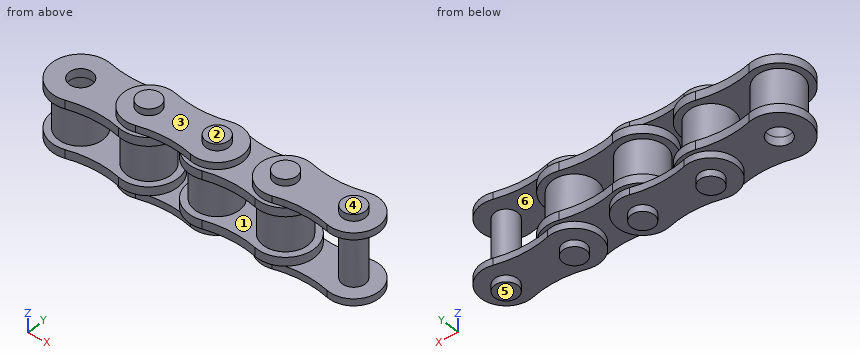
```python
from build123d import *

# Parameters (mm, degrees)
SKETCH4_R                  = 3.175
SKETCH4_R_2                = 1.6637
BOSS_EXTRUDE1_DEPTH        = 2.86
BOSS_EXTRUDE1_2_DEPTH      = 2.86
SKETCH5_R                  = 1.6383
BOSS_EXTRUDE2_DEPTH        = 1.2446
LPATTERN1_COUNT            = 2
LPATTERN1_PITCH            = 9.525
SKETCH7_R                  = 1.6383
BOSS_EXTRUDE3_DEPTH        = 0.9906
BOSS_EXTRUDE4_DEPTH        = 6.096
BOSS_EXTRUDE4_DEPTH_BACK   = 6.096
SKETCH8_R                  = 1.6383
BOSS_EXTRUDE4_2_DEPTH      = 6.096
BOSS_EXTRUDE4_2_DEPTH_BACK = 6.096
LPATTERN2_COUNT            = 2
LPATTERN2_PITCH            = 19.05


with BuildPart() as part:
    # Sketch4 → Boss-Extrude1 (new, symmetric)
    with BuildSketch(Plane.XY):
        with Locations((-4.7625, 0)):
            Circle(SKETCH4_R)
        with Locations((-4.7625, 0)):
            Circle(SKETCH4_R_2, mode=Mode.SUBTRACT)
    extrude(amount=BOSS_EXTRUDE1_DEPTH, both=True)


with BuildPart() as body_2:
    # Sketch4 → Boss-Extrude1 2 (new, symmetric)
    with BuildSketch(Plane.XY):
        with Locations((4.7625, 0)):
            Circle(SKETCH4_R)
        with Locations((4.7625, 0)):
            Circle(SKETCH4_R_2, mode=Mode.SUBTRACT)
    extrude(amount=BOSS_EXTRUDE1_2_DEPTH, both=True)


with BuildPart() as body_3:
    # Sketch5 → Boss-Extrude2 (new body)
    with BuildSketch(Plane.XY.offset(2.86)):
        with BuildLine():
            ThreePointArc((-3.71992076, 3.967398762), (-8.8646, 0), (-3.71992076, -3.967398762))
            ThreePointArc((-3.71992076, -3.967398762), (0, -3.486785), (3.71992076, -3.967398762))
            ThreePointArc((3.71992076, -3.967398762), (8.8646, 0), (3.71992076, 3.967398762))
            ThreePointArc((3.71992076, 3.967398762), (0, 3.486785), (-3.71992076, 3.967398762))
        make_face()
        with Locations((-4.7625, 0)):
            Circle(SKETCH5_R, mode=Mode.SUBTRACT)
        with Locations((4.7625, 0)):
            Circle(SKETCH5_R, mode=Mode.SUBTRACT)
    extrude(amount=BOSS_EXTRUDE2_DEPTH)


with BuildPart() as lpattern1_1:
    # LPattern1: pattern copy
    add(body_2.part.moved(Location(Vector(1, 0, 0) * (1 * LPATTERN1_PITCH))))


with BuildPart() as body_5:
    # Sketch7 → Boss-Extrude3 (new body)
    with BuildSketch(Plane.XY.offset(-4.1554)):
        with BuildLine():
            ThreePointArc((5.704721623, 3.48471247), (1.152652, 0), (5.704721623, -3.48471247))
            ThreePointArc((5.704721623, -3.48471247), (9.525, -2.977345042), (13.345278377, -3.48471247))
            ThreePointArc((13.345278377, -3.48471247), (17.897348, 0), (13.345278377, 3.48471247))
            ThreePointArc((13.345278377, 3.48471247), (9.525, 2.977345042), (5.704721623, 3.48471247))
        make_face()
        with Locations((4.7625, 0)):
            Circle(SKETCH7_R, mode=Mode.SUBTRACT)
        with Locations((14.2875, 0)):
            Circle(SKETCH7_R, mode=Mode.SUBTRACT)
    extrude(amount=-BOSS_EXTRUDE3_DEPTH)


with BuildPart() as body_6:
    # Mirror1: mirrored copy
    add(body_3.part.mirror(Plane.XY))


with BuildPart() as body_7:
    # Mirror1 2: mirrored copy
    add(body_5.part.mirror(Plane.XY))


with BuildPart() as body_8:
    # Sketch8 → Boss-Extrude4 (new, two sides: drawn at the far end of the back side and taken through both)
    with BuildSketch(Plane.XY.offset(-BOSS_EXTRUDE4_DEPTH_BACK)):
        with Locations(Location((4.7625, 0, 0), (0, 0, 180))):
            Circle(SKETCH8_R)
    extrude(amount=BOSS_EXTRUDE4_DEPTH + BOSS_EXTRUDE4_DEPTH_BACK)


with BuildPart() as body_9:
    # Sketch8 → Boss-Extrude4 2 (new, two sides: drawn at the far end of the back side and taken through both)
    with BuildSketch(Plane.XY.offset(-BOSS_EXTRUDE4_2_DEPTH_BACK)):
        with Locations(Location((14.2875, 0, 0), (0, 0, 180))):
            Circle(SKETCH8_R)
    extrude(amount=BOSS_EXTRUDE4_2_DEPTH + BOSS_EXTRUDE4_2_DEPTH_BACK)


with BuildPart() as lpattern2_1:
    # LPattern2: pattern copy
    add(body_9.part.moved(Location(Vector(1, 0, 0) * (1 * LPATTERN2_PITCH))))


with BuildPart() as lpattern2_2:
    # LPattern2: pattern copy
    add(body_8.part.moved(Location(Vector(1, 0, 0) * (1 * LPATTERN2_PITCH))))


with BuildPart() as lpattern2_3:
    # LPattern2: pattern copy
    add(body_7.part.moved(Location(Vector(1, 0, 0) * (1 * LPATTERN2_PITCH))))


with BuildPart() as lpattern2_4:
    # LPattern2: pattern copy
    add(body_6.part.moved(Location(Vector(1, 0, 0) * (1 * LPATTERN2_PITCH))))


with BuildPart() as lpattern2_5:
    # LPattern2: pattern copy
    add(body_5.part.moved(Location(Vector(1, 0, 0) * (1 * LPATTERN2_PITCH))))


with BuildPart() as lpattern2_6:
    # LPattern2: pattern copy
    add(lpattern1_1.part.moved(Location(Vector(1, 0, 0) * (1 * LPATTERN2_PITCH))))


with BuildPart() as lpattern2_7:
    # LPattern2: pattern copy
    add(body_3.part.moved(Location(Vector(1, 0, 0) * (1 * LPATTERN2_PITCH))))


with BuildPart() as lpattern2_8:
    # LPattern2: pattern copy
    add(body_2.part.moved(Location(Vector(1, 0, 0) * (1 * LPATTERN2_PITCH))))


with BuildPart() as lpattern2_9:
    # LPattern2: pattern copy
    add(part.part.moved(Location(Vector(1, 0, 0) * (1 * LPATTERN2_PITCH))))


with BuildPart() as body_2_1:
    add(body_2.part)

    # Combine1: union body 3, LPattern1_1, body 5, body 6, body 7, body 8, body 9, LPattern2_1, LPattern2_2, LPattern2_3, LPattern2_4, LPattern2_5, LPattern2_7, LPattern2_8, LPattern2_9, part
    add(body_3.part)
    add(lpattern1_1.part)
    add(body_5.part)
    add(body_6.part)
    add(body_7.part)
    add(body_8.part)
    add(body_9.part)
    add(lpattern2_1.part)
    add(lpattern2_2.part)
    add(lpattern2_3.part)
    add(lpattern2_4.part)
    add(lpattern2_5.part)
    add(lpattern2_7.part)
    add(lpattern2_8.part)
    add(lpattern2_9.part)
    add(part.part)


solid = body_2_1.part
```
The listing builds one solid part. Answer for the finished solid, in the listing's coordinates (mm). Face numbers are marked on the shaded views. A direction names the side the tool comes from. Round coordinates to 2 decimals unless told otherwise and drop trailing zeros. Loops run counter-clockwise (first coordinate to the right, second up) from the corner with the lowest first, then second, coordinate; pieces in that order, holes last. Notation, with made-up numbers: (86, 87) -> (105, 87) arc R22 ccw to (105, 97) -> close; hole circle Ø1 at (38.5, 85). An arc over 180 degrees is marked (long way). Use one line per item in the form item = value.
1. A tool of negligible diameter and unlimited length cuts with its end or side. For the marked faces 1, 2 and 3, from which of +Z, -Z, +X, -X, +Y, -Y can it reach the whole face along a straight path? Write none if from no direction.
Answer key:
face_1 = none
face_2 = +Z, +X, -X, +Y, -Y
face_3 = +Z
2. The part is cut by section D-D on x = 7.5. Determine the outline of the cut face in (y, z), and give its area (3 significant figures).
Answer key:
outline = (-3.12, -5.15) -> (3.12, -5.15) -> (3.12, -4.16) -> (-3.12, -4.16) -> close; (-3.12, 4.16) -> (3.12, 4.16) -> (3.12, 5.15) -> (-3.12, 5.15) -> close; (-3.06, -4.1) -> (3.06, -4.1) -> (3.06, -2.86) -> (1.61, -2.86) -> (1.61, 2.86) -> (3.06, 2.86) -> (3.06, 4.1) -> (-3.06, 4.1) -> (-3.06, 2.86) -> (-1.61, 2.86) -> (-1.61, -2.86) -> (-3.06, -2.86) -> close
area = 46.0 mm²
3. For a pull along Z with two mould halves and no side action, classify the marked faces 4, 5 and 6 as released by +Z, released by -Z, zero draft, split by the parting line, or undercut.
Answer key:
face_4 = released by +Z
face_5 = released by -Z
face_6 = undercut
4. Flat-ended cylindrical pins translate along their axes: pin 1 Ø3 at (y, z) = (2, -0.5) entering from -X; pin 2 Ø1.5 at (x, y) = (27.5, 3) entering from +Z; pin 3 Ø3.5 at (x, y) = (30, -1) entering from -Z. Find the tip coordinate at first contact, or state that the pin passes through.
Answer key:
pin_1 = -7.9
pin_2 = 5.15
pin_3 = -5.15
5. The part is cut by section A-A on z = 0.75. Give the number of separate pieces and of enclosed holes in the cut face, and give its area (3 significant figures).
Answer key:
separate_pieces = 8
enclosed_holes = 4
area = 126 mm²
6. Find the intervals of material crossed by probe 1 along X at (y, z) = (1.5, 3.5); probe 2 along Z at (x, y) = (18, 1.5); probe 3 along X at (y, z) = (-1, -3.75), in increasing order. Write a range as [from, to].
Answer key:
probe_1 = [-8.58, -5.42], [-4.1, 8.58], [10.47, 27.63], [32.68, 34]
probe_2 = [-4.1, -2.86], [2.86, 4.1]
probe_3 = [-8.74, -6.06], [-3.46, 8.74], [10.31, 27.79], [32.04, 34.64]
